Read the model definition and answer for the solid it produces. Units are mm, in the model's axes. Coordinates: 2 decimals unless noted, no trailing zeros. Write each loop counter-clockwise with the first axis right and the second up, starting at its lowest first coordinate (ties: lowest second). Pieces come first, ordered by that corner, then holes. Notation, with made-up numbers: (-33.75, 11.5) -> (-5.75, 11.5) arc R11 cw to (-5.75, 27.5) -> close; hole circle Ø1 at (-35.5, 61). An arc over 180 degrees is marked (long way). Answer as a JSON object with one key per item and string values. Group by question number.
(1) Find section B-B (z = 79.1). Give the vertices of the cut face in (x, y), then the cut area to 3 significant figures.
(2) Straight lines are drawn through the part: L1, parallel to Y at x = -110, z = 79.55; L2, parallel to X at y = -10, z = 80.2; L3, parallel to X at y = 8, z = 83.2. For each, find the intervals that lie inside material, in ascending order.
(3) For a pull along X with two mould halves and no side action, classify faces 1 (the face through (-107.615, -9.249, 80.958)), 2 (the face through (-92, -11.5, 81)), 3 (the face through (-74, 16, 81)), 4 (the face through (-122, -2, 81)) as +X half, -X half, draft (parallel to the pull), parting line (faces both ways), or undercut.
(4) Find section A-A (x = -90). Give the vertices of the cut face in (y, z).
(5) Find section C-C (y = -10). Give the vertices of the cut face in (x, z), then the cut area to 3 significant figures.
(6) Find section D-D (x = -111). Give the vertices of the cut face in (y, z).
from build123d import *

# Parameters (mm, degrees)
BOX749_W           = 148
BOX749_H           = 74
BOX749_DEPTH       = 55
CYLINDER1788_R     = 2.5
CYLINDER1788_DEPTH = 20
CYLINDER1789_R     = 2.5
CYLINDER1789_DEPTH = 20
CYLINDER1787_R     = 74
CYLINDER1787_DEPTH = 32
BOX748_W           = 62
BOX748_H           = 56
BOX748_DEPTH       = 6
CHAMFER062_SIZE    = 12


with BuildPart() as krychle749:
    # Box749 → Box749 (new body)
    with BuildSketch(Plane(origin=(-74, 0, 29), x_dir=(1, 0, 0), z_dir=(0, 0, 1))):
        with Locations((74, 37)):
            Rectangle(BOX749_W, BOX749_H)
    extrude(amount=BOX749_DEPTH)


with BuildPart() as obj1:
    # Cylinder1788 → Cylinder1788 (new body)
    with BuildSketch(Plane(origin=(-90, -10, 66), x_dir=(1, 0, 0), z_dir=(0, 0, 1))):
        Circle(CYLINDER1788_R)
    extrude(amount=CYLINDER1788_DEPTH)


with BuildPart() as compound914:
    # Cylinder1789 → Cylinder1789 (new body)
    with BuildSketch(Plane(origin=(-110, -10, 66), x_dir=(1, 0, 0), z_dir=(0, 0, 1))):
        Circle(CYLINDER1789_R)
    extrude(amount=CYLINDER1789_DEPTH)

    # Compound914: union obj1
    add(obj1.part)


with BuildPart() as obj2:
    # Cylinder1787 → Cylinder1787 (new body)
    with BuildSketch(Plane.XY.offset(66)):
        Circle(CYLINDER1787_R)
    extrude(amount=CYLINDER1787_DEPTH)


with BuildPart() as cut552:
    # Box748 → Box748 (new body)
    with BuildSketch(Plane(origin=(-122, -24, 76), x_dir=(1, 0, 0), z_dir=(0, 0, 1))):
        with Locations((31, 28)):
            Rectangle(BOX748_W, BOX748_H)
    extrude(amount=BOX748_DEPTH)

    # Cut545: cut obj2
    add(obj2.part, mode=Mode.SUBTRACT)

    # Cut544: cut Compound914
    add(compound914.part, mode=Mode.SUBTRACT)


with BuildPart() as cut552_1:
    # Cut544 placement: moved
    add(cut552.part.moved(Location((0, 0, 2))))

    # Chamfer062
    chamfer062_edges = [cut552_1.edges().sort_by_distance(p)[0] for p in [
        (-122, 32, 81),
    ]]
    chamfer(chamfer062_edges, length=CHAMFER062_SIZE)

    # Cut552: cut Krychle749
    add(krychle749.part, mode=Mode.SUBTRACT)


solid = cut552_1.part
Results below:
{
 "1": {"outline": "(-122, -24) -> (-70, -24) arc R74 cw to (-74, 0) -> (-74, 32) -> (-110, 32) -> (-122, 20) -> close; hole circle Ø5 at (-110, -10); hole circle Ø5 at (-90, -10)", "area": "2,610 mm2"},
 "2": {"L1": "y = -24 to -12.5, -7.5 to 32", "L2": "x = -122 to -112.5, -107.5 to -92.5, -87.5 to -73.32", "L3": "x = -122 to -74"},
 "3": {"face 1": "undercut", "face 2": "undercut", "face 3": "+X half", "face 4": "-X half"},
 "4": {"outline": "(-24, 78) -> (-12.5, 78) -> (-12.5, 84) -> (-24, 84) -> close; (-7.5, 78) -> (32, 78) -> (32, 84) -> (-7.5, 84) -> close"},
 "5": {"outline": "(-122, 78) -> (-112.5, 78) -> (-112.5, 84) -> (-122, 84) -> close; (-107.5, 78) -> (-92.5, 78) -> (-92.5, 84) -> (-107.5, 84) -> close; (-87.5, 78) -> (-73.32, 78) -> (-73.32, 84) -> (-87.5, 84) -> close", "area": "232 mm2"},
 "6": {"outline": "(-24, 78) -> (-12.29, 78) -> (-12.29, 84) -> (-24, 84) -> close; (-7.71, 78) -> (31, 78) -> (31, 84) -> (-7.71, 84) -> close"}
}
